```python
from build123d import *

# Parameters (mm, degrees)
F0_W      = 38.1
F0_H      = 38.1
F1_DEPTH  = 736.6
F2_W      = 38.1
F2_H      = 38.1
F3_DEPTH  = 368.3
F4_W      = 38.1
F4_H      = 38.1
F5_DEPTH  = 736.6
F6_W      = 38.1
F6_H      = 38.1
F7_DEPTH  = 368.3
F8_W      = 101.6
F8_H      = 368.3
F9_DEPTH  = 19.05
F10_W     = 101.6
F10_H     = 368.3
F11_DEPTH = 19.05
F12_W     = 114.3
F12_H     = 368.3
F13_DEPTH = 19.0246
F14_W     = 114.3
F14_H     = 368.3
F15_DEPTH = 19.0246
F16_W     = 177.8
F16_H     = 444.5
F16_W_2   = 152.4
F16_H_2   = 368.3
F17_DEPTH = 19.05


with BuildPart() as f1:
    # F0 (on Right) → F1 (new body)
    with BuildSketch(Plane.YZ):
        with Locations((-19.05, -19.05)):
            Rectangle(F0_W, F0_H)
    extrude(amount=F1_DEPTH)

    # F2 (on face) → F3 (join)
    with BuildSketch(Plane(origin=(0, 0, 0), x_dir=(-1, 0, 0), z_dir=(0, 1, 0))):
        with Locations((-19.05, -19.05)):
            Rectangle(F2_W, F2_H)
        with Locations((-717.55, -19.05)):
            Rectangle(F2_W, F2_H)
    extrude(amount=F3_DEPTH)

    # F4 (on face) → F5 (join)
    with BuildSketch(Plane.YZ.offset(736.6)):
        with Locations((387.35, -19.05)):
            Rectangle(F4_W, F4_H)
    extrude(amount=-F5_DEPTH)

    # F6 (on face) → F7 (join, through all)
    with BuildSketch(Plane.XZ.offset(-368.3)):
        with Locations((273.05, -19.05)):
            Rectangle(F6_W, F6_H)
        with Locations((463.55, -19.05)):
            Rectangle(F6_W, F6_H)
    extrude(amount=F7_DEPTH)

    # F8 (on face) → F9 (join)
    with BuildSketch(Plane.XY):
        Polygon((139.7, 406.4), (0, 406.4), (0, -38.1), (139.7, -38.1), (139.7, 0), (38.1, 0), (38.1, 368.3), (139.7, 368.3), align=None)
        with Locations((88.9, 184.15)):
            Rectangle(F8_W, F8_H)
    extrude(amount=F9_DEPTH)

    # F10 (on face) → F11 (join)
    with BuildSketch(Plane.XY):
        with Locations((647.7, 184.15)):
            Rectangle(F10_W, F10_H)
        Polygon((736.6, -38.1), (736.6, 406.4), (596.9, 406.4), (596.9, 368.3), (698.5, 368.3), (698.5, 0), (596.9, 0), (596.9, -38.1), align=None)
    extrude(amount=F11_DEPTH)

    # F12 (on face) → F13 (join)
    with BuildSketch(Plane.XY):
        Polygon((279.4, 406.4), (139.7, 406.4), (139.7, 368.3), (254, 368.3), (254, 0), (139.7, 0), (139.7, -38.1), (279.4, -38.1), align=None)
        with Locations((196.85, 184.15)):
            Rectangle(F12_W, F12_H)
    extrude(amount=F13_DEPTH)

    # F14 (on face) → F15 (join)
    with BuildSketch(Plane.XY):
        Polygon((596.9, 368.3), (596.9, 406.4), (457.2, 406.4), (457.2, -38.1), (596.9, -38.1), (596.9, 0), (482.6, 0), (482.6, 368.3), align=None)
        with Locations((539.75, 184.15)):
            Rectangle(F14_W, F14_H)
    extrude(amount=F15_DEPTH)

    # F16 (on face) → F17 (join)
    with BuildSketch(Plane.XY):
        with Locations((368.3, 184.15)):
            Rectangle(F16_W, F16_H)
        with Locations((368.3, 184.15)):
            Rectangle(F16_W_2, F16_H_2, mode=Mode.SUBTRACT)
        with Locations((368.3, 184.15)):
            Rectangle(F16_W_2, F16_H_2)
    extrude(amount=F17_DEPTH)


solid = f1.part
```
For this review, take the finished solid that the model builds, in its own axes (mm). A direction names the side the tool comes from. Round coordinates to 2 decimals unless told otherwise and drop trailing zeros. Write each loop counter-clockwise with the first axis right and the second up, starting at its lowest first coordinate (ties: lowest second). Pieces come first, ordered by that corner, then holes. Notation, with made-up numbers: (40.5, -21.5) -> (80.5, -21.5) arc R16 ccw to (80.5, -17.5) -> close; hole circle Ø9 at (12, 23). An arc over 180 degrees is marked (long way). One line per question, with ' | ' between items. Start each with the question number.
1) Machinability: for faces 1 (the flat face through (455, 181, -38.1)), 2 (the flat face through (698.5, 182, -19)), which of the approach directions +Z, -Z, +X, -X, +Y, -Y give a long, thin tool a straight path to every point of the face, cutting with its end or side? Answer none if there is none.
2) Mouldability with a two-part tool opening along X and no side actions: class faces 3 (the flat face through (145, 187, 0)), 4 (the flat face through (0, 187, -10)), 5 (the flat face through (363, -38.1, -10)) as +X half, -X half, draft (parallel to the pull), parting line (faces both ways), or undercut.
3) Add section A-A (x = 51.5). Write out the cut boundary in (y, z).
4) Add section B-B (z = -8.5). Write out the cut boundary in (x, y), and give its area (3 significant figures).
5) For pin 1 Ø11.5 at (y, z) = (199, -19.5) entering from -X; pin 2 Ø1 at (x, y) = (563.5, 143.5) entering from +Z; pin 3 Ø8 at (x, y) = (204.5, 54) entering from -Z, all flat-tipped, find the tip position at first contact; note any pin that passes through.
6) Wall thickness on line 1 along X through (y, z) = (361, -16); line 2 along Y through (x, z) = (697, -5); line 3 along Z through (x, y) = (209, 304.5): over which ranges is each line inside the solid? List them lowest first.
7) Add section D-D (x = 181.5). Write out the cut boundary in (y, z).
Reported:
1) face 1: -Z, +X, -X, +Y, -Y | face 2: -Z
2) face 3: undercut | face 4: -X half | face 5: draft
3) outline: (-38.1, -38.1) -> (0, -38.1) -> (0, 0) -> (368.3, 0) -> (368.3, -38.1) -> (406.4, -38.1) -> (406.4, 19.05) -> (-38.1, 19.05) -> close
4) outline: (0, -38.1) -> (736.6, -38.1) -> (736.6, 406.4) -> (0, 406.4) -> close; hole (38.1, 0) -> (254, 0) -> (254, 368.3) -> (38.1, 368.3) -> close; hole (292.1, 0) -> (444.5, 0) -> (444.5, 368.3) -> (292.1, 368.3) -> close; hole (482.6, 0) -> (698.5, 0) -> (698.5, 368.3) -> (482.6, 368.3) -> close | area: 112,000 mm²
5) pin 1: stops at x = 0 | pin 2: stops at z = 19.02 | pin 3: stops at z = 0
6) line 1: x = 0 to 38.1, 254 to 292.1, 444.5 to 482.6, 698.5 to 736.6 | line 2: y = -38.1 to 0, 368.3 to 406.4 | line 3: z = 0 to 19.02
7) outline: (-38.1, -38.1) -> (0, -38.1) -> (0, 0) -> (368.3, 0) -> (368.3, -38.1) -> (406.4, -38.1) -> (406.4, 19.02) -> (-38.1, 19.02) -> close
